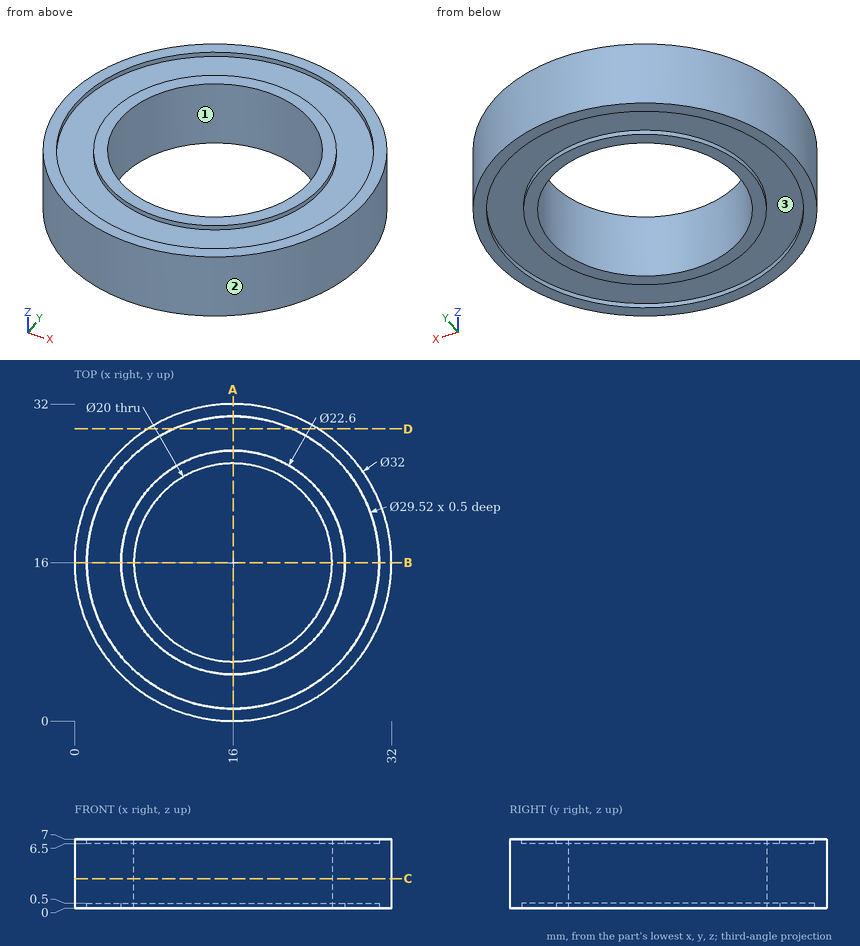
Print and shaded views of the part. All mm, measured from the part's lowest x, y and z. Give positions to 0.01 mm unless a question says otherwise; leave off trailing zeros. Order: outer loops, then holes, each group sorted by start corner. A loop starts at its lowest first (then second) coordinate and runs counter-clockwise, first axis right, second up. Notation, with made-up numbers: (50.5, 65) -> (60.5, 65) arc R31 cw to (60.5, 96) -> close; hole circle Ø10 at (45, 42). An arc over 180 degrees is marked (long way). Use CSV: the item, a comma, the result in double quotes.
1. Mould opens along X. For the marked faces 1, 2 and 3 say: +X half, -X half, draft (parallel to the pull), parting line (faces both ways), or undercut.
Outcome:
face 1,"undercut"
face 2,"parting line"
face 3,"undercut"
2. Band-saw the part on D-D, the plane y = 29.5. Give the cut face in (x, z), then the cut area to 3 significant figures.
Outcome:
outline,"(7.41, 0) -> (10.03, 0) -> (10.03, 0.5) -> (21.97, 0.5) -> (21.97, 0) -> (24.59, 0) -> (24.59, 7) -> (21.97, 7) -> (21.97, 6.5) -> (10.03, 6.5) -> (10.03, 7) -> (7.41, 7) -> close"
area,"108 mm²"
3. Drop flat-ended pins along their axis: pin 1 (9 mm diameter, centred on x = 17.5, y = 15, fed in from +Z); pin 2 (1 mm diameter, centred on x = 22, z = 3.5, fed in from +Y) (3 decimals); pin 3 (1.5 mm diameter, centred on x = 26, z = 5, fed in from -Y); pin 4 (1.5 mm diameter, centred on y = 13, z = 2.5, fed in from +X). Give the stop position or say it passes through.
Outcome:
pin 1,"through"
pin 2,"y = 31.025"
pin 3,"y = 2.94"
pin 4,"x = 31.84"
4. Band-saw the part on C-C, the plane z = 3. Give the cut face in (x, y), then the cut area to 3 significant figures.
Outcome:
outline,"circle Ø32 at (16, 16); hole circle Ø20 at (16, 16)"
area,"490 mm²"
5. Drill centre lines: line 1 along Y through (x, z) = (16, 0.35); line 2 along Y through (x, z) = (16, 3.25); line 3 along Z through (x, y) = (7, 25). Where is each one in solid material? Low to high. Write a range as from..to.
Outcome:
line 1,"0..1.24, 4.7..6, 26..27.3, 30.76..32"
line 2,"0..6, 26..32"
line 3,"0.5..6.5"
6. Band-saw the part on A-A, the plane x = 16. Give the cut face in (y, z), then the cut area to 3 significant figures.
Outcome:
outline,"(0, 0) -> (1.24, 0) -> (1.24, 0.5) -> (4.7, 0.5) -> (4.7, 0) -> (6, 0) -> (6, 7) -> (4.7, 7) -> (4.7, 6.5) -> (1.24, 6.5) -> (1.24, 7) -> (0, 7) -> close; (26, 0) -> (27.3, 0) -> (27.3, 0.5) -> (30.76, 0.5) -> (30.76, 0) -> (32, 0) -> (32, 7) -> (30.76, 7) -> (30.76, 6.5) -> (27.3, 6.5) -> (27.3, 7) -> (26, 7) -> close"
area,"77.1 mm²"
